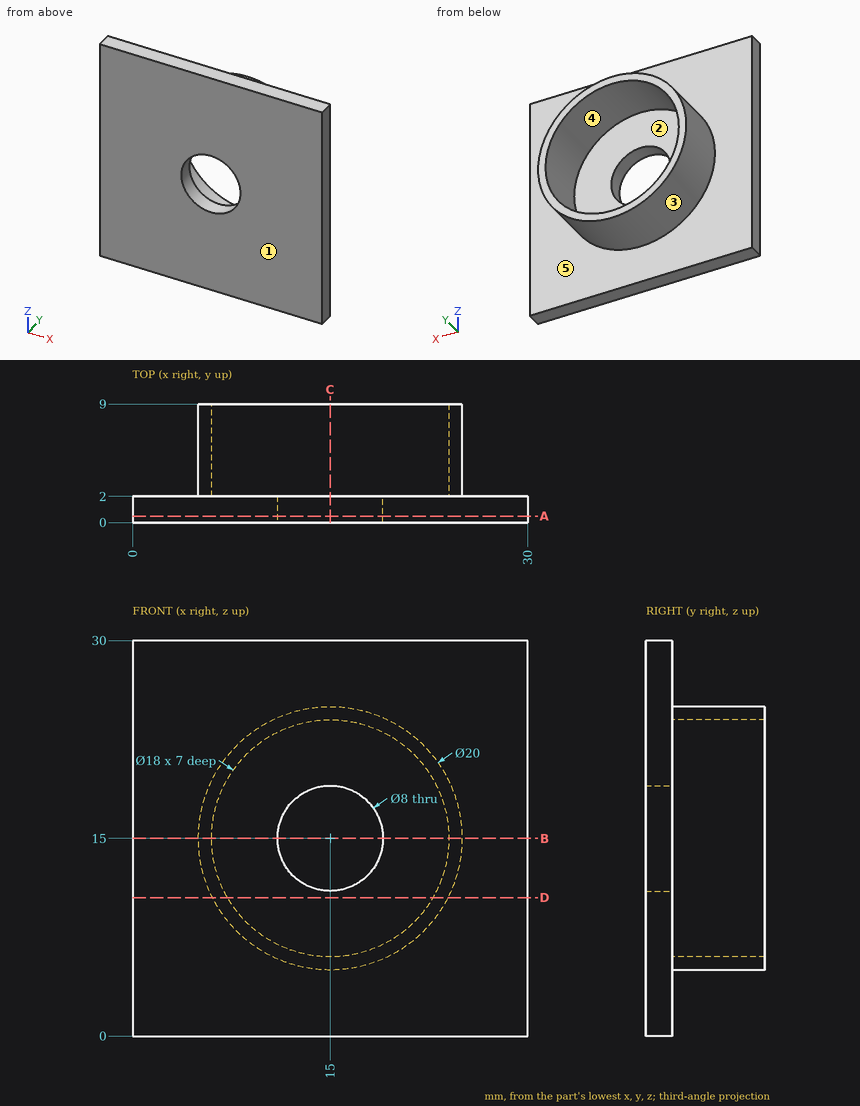
The figure shows three views and two pictorial views of one solid part (mm, origin at its lowest corner). Answer the questions. A direction names the side the tool comes from. Give positions to 0.01 mm unless a question says otherwise; leave off trailing zeros. Order: outer loops, then holes, each group sorted by start corner. A loop starts at its lowest first (then second) coordinate and runs counter-clockwise, first axis right, second up. Notation, with made-up numbers: (30, 1) -> (87, 1) arc R13 cw to (87, 16) -> close; hole circle Ø3 at (-28, -38.75). An arc over 180 degrees is marked (long way). Answer as CSV lines item,"result". Start each with the question number.
Q1. Determine the mould class of the marked faces 3, 4 and 5 for opening direction Z: pulls with the +Z half, pulls with the -Z half, needs draft (parallel to the pull), parting line crosses it, or undercut.
Q2. Given pin 1 (5.5 mm diameter, centred on x = 13, z = 11, fed in from +Y); pin 2 (1.5 mm diameter, centred on x = 23.5, y = 6, fed in from -Z); pin 3 (1.5 mm diameter, centred on x = 17, y = 4.5, fed in from +Z), each flat-ended and moving along its own axis, determine where each tip first touches the part or whether it passes through.
Q3. A cutting plane is placed at D-D (z = 10.5). Determine the outline of the cut face in (x, y).
Q4. Which of the six approach directions +Z, -Z, +X, -X, +Y, -Y give full straight-line access (tool end or side, diameter ignored) to the marked faces 1 and 2?
Q5. A cutting plane is placed at C-C (x = 15). Determine the outline of the cut face in (y, z), then the cut area to 3 significant figures.
Q6. Find the intervals of material crossed by L1, parallel to Z at x = 15, y = 0.6; L2, parallel to Z at x = 15, y = 7; L3, parallel to Y at x = 19.5, z = 5.25, in increasing order.
Q7. A cutting plane is placed at B-B (z = 15). Determine the outline of the cut face in (x, y).
Q8. A cutting plane is placed at A-A (y = 0.5). Determine the outline of the cut face in (x, z), then the cut area to 3 significant figures.
Results found:
1,face 3,"parting line crosses it"
1,face 4,"undercut"
1,face 5,"needs draft"
2,pin 1,"y = 2"
2,pin 2,"z = 8.68"
2,pin 3,"z = 24.92"
3,outline,"(0, 0) -> (30, 0) -> (30, 2) -> (23.93, 2) -> (23.93, 9) -> (22.79, 9) -> (22.79, 2) -> (7.21, 2) -> (7.21, 9) -> (6.07, 9) -> (6.07, 2) -> (0, 2) -> close"
4,face 1,"+Z, -Z, +X, -X, -Y"
4,face 2,"+Y"
5,outline,"(0, 0) -> (2, 0) -> (2, 5) -> (9, 5) -> (9, 6) -> (2, 6) -> (2, 11) -> (0, 11) -> close; (0, 19) -> (2, 19) -> (2, 24) -> (9, 24) -> (9, 25) -> (2, 25) -> (2, 30) -> (0, 30) -> close"
5,area,"58.0 mm2"
6,L1,"0 to 11, 19 to 30"
6,L2,"5 to 6, 24 to 25"
6,L3,"0 to 2"
7,outline,"(0, 0) -> (11, 0) -> (11, 2) -> (6, 2) -> (6, 9) -> (5, 9) -> (5, 2) -> (0, 2) -> close; (19, 0) -> (30, 0) -> (30, 2) -> (25, 2) -> (25, 9) -> (24, 9) -> (24, 2) -> (19, 2) -> close"
8,outline,"(0, 0) -> (30, 0) -> (30, 30) -> (0, 30) -> close; hole circle Ø8 at (15, 15)"
8,area,"850 mm2"
